```python
from build123d import *

# Parameters (mm, degrees)
BOSS_EXTRUDE1_REACH             = 25.885
BOSS_EXTRUDE1_DIRECTION_2_REACH = 25.885


with BuildPart() as part:
    # Sketch2 → Revolve1 (revolve)
    with BuildSketch(Plane.XY, mode=Mode.PRIVATE) as revolve1_sk:
        Polygon((-22.5552, 0), (-22.5552, 3.175), (-1.9812, 3.175), (-1.9812, 5.55625), (1.9812, 5.55625), (1.9812, 3.175), (22.5552, 3.175), (22.5552, 0), align=None)
    revolve(revolve1_sk.sketch.rotate(Axis((-22.5552, 0, 0), (1, 0, 0)), 90), axis=Axis((-22.5552, 0, 0), (1, 0, 0)))

    # Boss-Extrude1: up to this face of the body (flat: up to its plane)
    boss_extrude1_end = Plane(part.part.faces().sort_by_distance((1.9812, 0, -5.399095518))[0])
    # Sketch3 → Boss-Extrude1 (add, up to the picked face)
    with BuildSketch(Plane(origin=(0, 0, 0), x_dir=(0, 0, -1), z_dir=(1, 0, 0)), mode=Mode.PRIVATE) as boss_extrude1_sk1:
        Polygon((3.207902433, -5.55625), (6.415804866, 0), (3.207902433, 5.55625), (-3.207902433, 5.55625), (-6.415804866, 0), (-3.207902433, -5.55625), align=None)
    boss_extrude1_tool1 = split(extrude(boss_extrude1_sk1.sketch, amount=BOSS_EXTRUDE1_REACH, mode=Mode.PRIVATE), bisect_by=boss_extrude1_end, keep=Keep.BOTH, mode=Mode.PRIVATE)
    add(boss_extrude1_tool1.solids().sort_by(Axis((0, 0, 0), (1, 0, 0)))[0])

    # Boss-Extrude1 direction 2: up to this face of the body (flat: up to its plane)
    boss_extrude1_direction_2_end = Plane(part.part.faces().sort_by_distance((-1.9812, 0, -3.332154482))[0])
    # Sketch3 → Boss-Extrude1 direction 2 (add, up to the picked face)
    with BuildSketch(Plane(origin=(0, 0, 0), x_dir=(0, 0, -1), z_dir=(1, 0, 0)), mode=Mode.PRIVATE) as boss_extrude1_direction_2_sk1:
        Polygon((3.207902433, -5.55625), (6.415804866, 0), (3.207902433, 5.55625), (-3.207902433, 5.55625), (-6.415804866, 0), (-3.207902433, -5.55625), align=None)
    boss_extrude1_direction_2_tool1 = split(extrude(boss_extrude1_direction_2_sk1.sketch, amount=-BOSS_EXTRUDE1_DIRECTION_2_REACH, mode=Mode.PRIVATE), bisect_by=boss_extrude1_direction_2_end, keep=Keep.BOTH, mode=Mode.PRIVATE)
    add(boss_extrude1_direction_2_tool1.solids().sort_by(Axis((0, 0, 0), (-1, 0, 0)))[0])


solid = part.part
```
Geometry: final body of the model. Coordinates: model frame, mm. A direction names the side the tool comes from. Give positions to 0.01 mm unless a question says otherwise; leave off trailing zeros. Loops run counter-clockwise (first coordinate to the right, second up) from the corner with the lowest first, then second, coordinate; pieces in that order, holes last. Notation, with made-up numbers: (50, 19.5) -> (92, 19.5) arc R28 cw to (92, 56.5) -> close; hole circle Ø8 at (-22, 84.5). An arc over 180 degrees is marked (long way). Use one line per item in the form item = value.
Item 1: Access query for faces 1 (the face through (1.981, -3, 3)), 2 (the face through (-0.028, 2.739, -4.834)), 3 (the face through (-1.981, -3, -3)). Directions: +Z, -Z, +X, -X, +Y, -Y. A direction counts if a zero-diameter tool reaches every point of the face in a straight line with its end or side. Return the directions, or none.
A:
face_1 = +X
face_2 = -Z, +X, -X, +Y
face_3 = -X
Item 2: Section query B-B on y = 0.75. Output: boundary loops of the cut face in (x, z), and give its area (3 significant figures).
A:
outline = (-22.56, -3.09) -> (-1.98, -3.09) -> (-1.98, -5.98) -> (1.98, -5.98) -> (1.98, -3.09) -> (22.56, -3.09) -> (22.56, 3.09) -> (1.98, 3.09) -> (1.98, 5.98) -> (-1.98, 5.98) -> (-1.98, 3.09) -> (-22.56, 3.09) -> close
area = 301 mm^2
Item 3: Line query: probe 1 along X at (y, z) = (0.25, 3.75); probe 2 along Z at (x, y) = (-8.5, -0.25); probe 3 along Y at (x, z) = (3, -1). Output: solid intervals per line, ascending.
A:
probe_1 = -1.98 to 1.98
probe_2 = -3.17 to 3.17
probe_3 = -3.01 to 3.01
Item 4: Section query C-C on x = 1. Output: boundary loops of the cut face in (y, z).
A:
outline = (-5.56, -3.21) -> (0, -6.42) -> (5.56, -3.21) -> (5.56, 3.21) -> (0, 6.42) -> (-5.56, 3.21) -> close
Item 5: Section query A-A on z = 0. Output: boundary loops of the cut face in (x, y) (3 decimals).
A:
outline = (-22.555, -3.175) -> (-1.981, -3.175) -> (-1.981, -5.556) -> (1.981, -5.556) -> (1.981, -3.175) -> (22.555, -3.175) -> (22.555, 3.175) -> (1.981, 3.175) -> (1.981, 5.556) -> (-1.981, 5.556) -> (-1.981, 3.175) -> (-22.555, 3.175) -> close
Item 6: Section query D-D on x = 16. Output: boundary loops of the cut face in (y, z) (3 decimals), and give its area (3 significant figures).
A:
outline = circle Ø6.35 at (0, 0)
area = 31.7 mm^2
Item 7: Pin query (flat end, axial travel): P1, Ø2, axis at x = -7.5, y = -0.5, coming from the +Z side (3 decimals); P2, Ø2, axis at x = -6.5, z = -2.5, coming from the -Y side. Return the tip coordinate at first contact, or that it passes through.
A:
P1 = 3.175
P2 = -2.8
